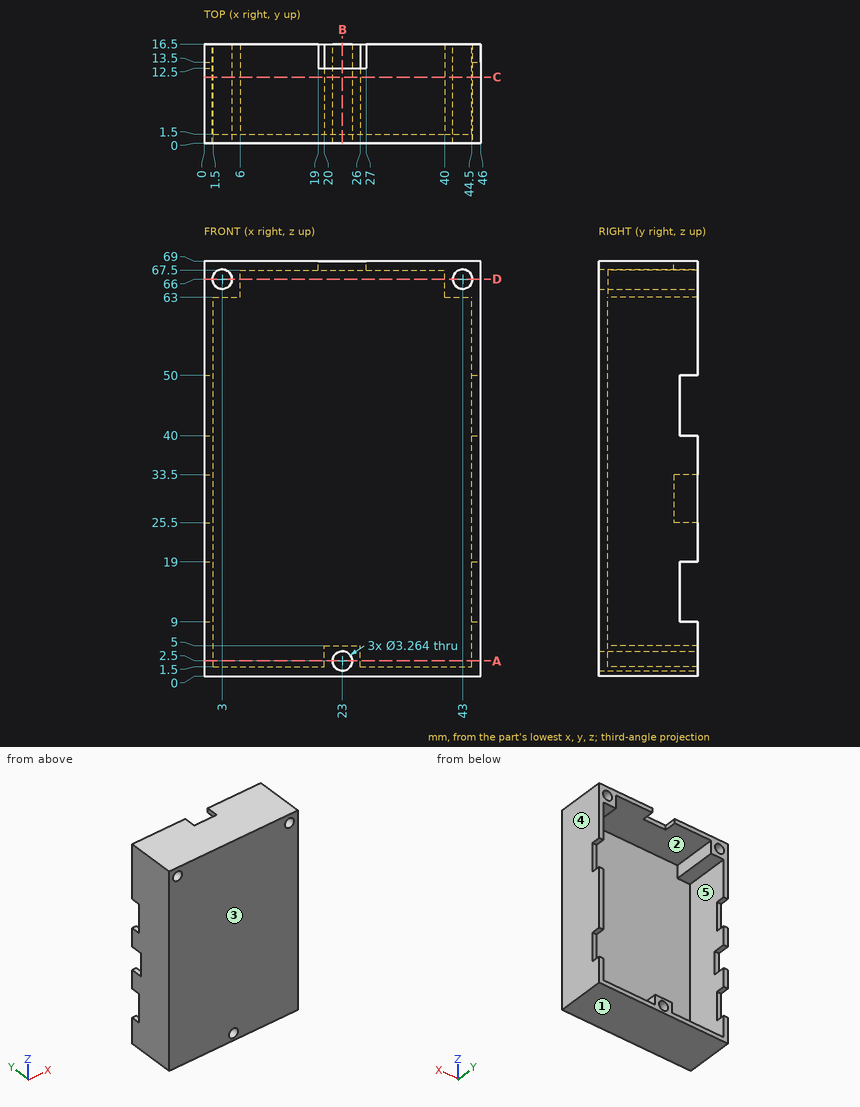
Geometry check sheet. Reference: drawing and pictorial views, mm from the part's lowest x, y, z. A direction names the side the tool comes from. Round coordinates to 2 decimals unless told otherwise and drop trailing zeros. Order: outer loops, then holes, each group sorted by start corner. A loop starts at its lowest first (then second) coordinate and runs counter-clockwise, first axis right, second up. Notation, with made-up numbers: (-3, 38.5) - (52, 38.5) arc R12 ccw to (52, 61.5) - close; hole circle Ø6 at (34, 44.25). An arc over 180 degrees is marked (long way). One line per question, with ' | ' between items. Start each with the question number.
(1) Depth check by flat-ended pin: pin 1 Ø0.8 at (y, z) = (14.5, 68.5) entering from -X; pin 2 Ø1.2 at (x, z) = (45.5, 46) entering from +Y. Enter the tip coordinate at first touch or a pass-through.
(2) Thickness scan on L1, parallel to X at y = 12.25, z = 66; L2, parallel to Z at x = 23, y = 11.5; L3, parallel to Z at x = 3, y = 7. Record the ranges inside material, lowest first. Write a range as [from, to].
(3) Release check for a two-part mould opening along Z. For the marked faces 1, 2 and 3 record: released by +Z, released by -Z, zero draft, split by the parting line, or undercut.
(4) Sectioned sample at D-D on z = 66. Record the cut outline in (x, y), and give its area (3 significant figures).
(5) Sectioned sample at B-B on x = 23. Record the cut outline in (y, z), and give its area (3 significant figures).
(6) Sectioned sample at C-C on y = 11. Record the cut outline in (x, z), and give its area (3 significant figures).
(7) Access from +Z, -Z, +X, -X, +Y, -Y to the whole of each face (thin tool, end or side, straight path). Record for the marked faces 4 and 5.
(8) Sectioned sample at A-A on z = 2.5. Record the cut outline in (x, y), and give its area (3 significant figures).
Conclusion:
1) pin 1: stops at x = 0 | pin 2: stops at y = 13.5
2) L1: x = [0, 1.37], [4.63, 6], [40, 41.37], [44.63, 46] | L2: z = [0, 0.87], [4.13, 5], [67.5, 69] | L3: z = [0, 1.5], [63, 64.37], [67.63, 69]
3) face 1: released by -Z | face 2: undercut | face 3: zero draft
4) outline: (0, 0) - (1.37, 0) - (1.37, 16.5) - (0, 16.5) - close; (4.63, 0) - (41.37, 0) - (41.37, 16.5) - (40, 16.5) - (40, 1.5) - (6, 1.5) - (6, 16.5) - (4.63, 16.5) - close; (44.63, 0) - (46, 0) - (46, 16.5) - (44.63, 16.5) - close | area: 141 mm2
5) outline: (0, 0) - (16.5, 0) - (16.5, 0.87) - (0, 0.87) - close; (0, 4.13) - (16.5, 4.13) - (16.5, 5) - (1.5, 5) - (1.5, 67.5) - (12.5, 67.5) - (12.5, 69) - (0, 69) - close | area: 141 mm2
6) outline: (0, 0) - (46, 0) - (46, 69) - (0, 69) - close; hole circle Ø3.26 at (3, 66); hole (1.5, 1.5) - (20, 1.5) - (20, 5) - (26, 5) - (26, 1.5) - (44.5, 1.5) - (44.5, 63) - (40, 63) - (40, 67.5) - (6, 67.5) - (6, 63) - (1.5, 63) - close; hole circle Ø3.26 at (23, 2.5); hole circle Ø3.26 at (43, 66) | area: 372 mm2
7) face 4: +Z, -Z, +X, +Y, -Y | face 5: +Y
8) outline: (0, 0) - (21.37, 0) - (21.37, 16.5) - (20, 16.5) - (20, 1.5) - (1.5, 1.5) - (1.5, 16.5) - (0, 16.5) - close; (24.63, 0) - (46, 0) - (46, 16.5) - (44.5, 16.5) - (44.5, 1.5) - (26, 1.5) - (26, 16.5) - (24.63, 16.5) - close | area: 150 mm2
